```python
from build123d import *

# Parameters (mm, degrees)
SKETCH_1_W          = 403
SKETCH_1_H          = 40
EXTRUDE_1_DEPTH     = 2
CUT_EXTRUDE_1_DEPTH = 203.5
FILLET_1_R          = 1.5
SKETCH_3_R          = 2.1
SKETCH_3_R_2        = 1.6
SKETCH_3_R_3        = 2.6
CUT_EXTRUDE_2_DEPTH = 203.5


with BuildPart() as part:
    # 草图1 → 凸台-拉伸1 (new body)
    with BuildSketch(Plane.XY):
        Rectangle(SKETCH_1_W, SKETCH_1_H)
    extrude(amount=EXTRUDE_1_DEPTH)

    # 草图2 → 切除-拉伸1 (cut, through all)
    with BuildSketch(Plane.XY.offset(2)):
        Polygon((-157.550139231, -12), (-185, 8.270666414), (-185, -12), align=None)
        Polygon((-179.949860769, 12), (-155.5, -6.055281799), (-155.5, 12), align=None)
        Polygon((-149.5, 6.055281799), (-149.5, -12), (-125.050139231, -12), align=None)
        Polygon((-147.449860769, 12), (-123, -6.055281799), (-123, 12), align=None)
        Polygon((-87, 6.518202701), (-87, -12), (-58.06530828, -12), align=None)
        Polygon((-84.43469172, 12), (-55.5, -6.518202701), (-55.5, 12), align=None)
        Polygon((-46.93469172, 12), (-18, -6.518202701), (-18, 12), align=None)
        Polygon((-49.5, 6.518202701), (-49.5, -12), (-20.56530828, -12), align=None)
        Polygon((46.93469172, 12), (18, 12), (18, -6.518202701), align=None)
        Polygon((49.5, -12), (49.5, 6.518202701), (20.56530828, -12), align=None)
        Polygon((84.43469172, 12), (55.5, 12), (55.5, -6.518202701), align=None)
        Polygon((87, 6.518202701), (58.06530828, -12), (87, -12), align=None)
        Polygon((123, 12), (123, -6.055281799), (147.449860769, 12), align=None)
        Polygon((149.5, 6.055281799), (125.050139231, -12), (149.5, -12), align=None)
        Polygon((155.5, 12), (155.5, -6.055281799), (179.949860769, 12), align=None)
        Polygon((185, 8.270666414), (157.550139231, -12), (185, -12), align=None)
    extrude(amount=-CUT_EXTRUDE_1_DEPTH, mode=Mode.SUBTRACT)

    # 圆角1
    fillet_1_edges = [part.edges().sort_by_distance(p)[0] for p in [
        (-87, 6.518202701, 1),
        (-58.06530828, -12, 1),
        (-87, -12, 1),
        (149.5, 6.055281799, 1),
        (149.5, -12, 1),
        (125.050139231, -12, 1),
        (155.5, 12, 1),
        (179.949860769, 12, 1),
        (155.5, -6.055281799, 1),
        (185, 8.270666414, 1),
        (185, -12, 1),
        (157.550139231, -12, 1),
        (49.5, -12, 1),
        (20.56530828, -12, 1),
        (49.5, 6.518202701, 1),
        (84.43469172, 12, 1),
        (55.5, -6.518202701, 1),
        (55.5, 12, 1),
        (87, 6.518202701, 1),
        (87, -12, 1),
        (58.06530828, -12, 1),
        (123, 12, 1),
        (147.449860769, 12, 1),
        (123, -6.055281799, 1),
        (-157.550139231, -12, 1),
        (-185, -12, 1),
        (-185, 8.270666414, 1),
        (-84.43469172, 12, 1),
        (-55.5, 12, 1),
        (-55.5, -6.518202701, 1),
        (-46.93469172, 12, 1),
        (-18, 12, 1),
        (-18, -6.518202701, 1),
        (-49.5, 6.518202701, 1),
        (-20.56530828, -12, 1),
        (-49.5, -12, 1),
        (46.93469172, 12, 1),
        (18, -6.518202701, 1),
        (18, 12, 1),
        (-179.949860769, 12, 1),
        (-155.5, 12, 1),
        (-155.5, -6.055281799, 1),
        (-149.5, 6.055281799, 1),
        (-125.050139231, -12, 1),
        (-149.5, -12, 1),
        (-147.449860769, 12, 1),
        (-123, 12, 1),
        (-123, -6.055281799, 1),
    ]]
    fillet(fillet_1_edges, radius=FILLET_1_R)

    # 草图3 → 切除-拉伸2 (cut, through all)
    with BuildSketch(Plane(origin=(0, 0, 0), x_dir=(-1, 0, 0), z_dir=(0, 0, -1))):
        with Locations((195, -7.5)):
            Circle(SKETCH_3_R)
        with Locations((-195, 7.5)):
            Circle(SKETCH_3_R)
        with Locations((195, 7.5)):
            Circle(SKETCH_3_R)
        with Locations((105, 7.5)):
            Circle(SKETCH_3_R)
        with Locations((105, -7.5)):
            Circle(SKETCH_3_R)
        with Locations((-105, 7.5)):
            Circle(SKETCH_3_R)
        with Locations((-105, -7.5)):
            Circle(SKETCH_3_R)
        with Locations((-195, -7.5)):
            Circle(SKETCH_3_R)
        with Locations((-152.5, -14.5)):
            Circle(SKETCH_3_R_2)
        with Locations((-185, 14.5)):
            Circle(SKETCH_3_R_2)
        with Locations((-185, -14.5)):
            Circle(SKETCH_3_R_2)
        with Locations((185, -14.5)):
            Circle(SKETCH_3_R_2)
        with Locations((-52.5, -14.5)):
            Circle(SKETCH_3_R_2)
        with Locations((52.5, -14.5)):
            Circle(SKETCH_3_R_2)
        with Locations((152.5, -14.5)):
            Circle(SKETCH_3_R_2)
        with Locations((152.5, 14.5)):
            Circle(SKETCH_3_R_2)
        with Locations((185, 14.5)):
            Circle(SKETCH_3_R_2)
        with Locations((-152.5, 14.5)):
            Circle(SKETCH_3_R_2)
        with Locations((-52.5, 14.5)):
            Circle(SKETCH_3_R_2)
        with Locations((52.5, 14.5)):
            Circle(SKETCH_3_R_2)
        with Locations((0, -7.5)):
            Circle(SKETCH_3_R_3)
        with Locations((0, 7.5)):
            Circle(SKETCH_3_R_3)
        with BuildLine():
            Line((-57, 12), (-79.30828758, 12))
            ThreePointArc((-79.30828758, 12), (-80.7479248, 10.921241824), (-80.116868125, 9.236592899))
            Line((-80.116868125, 9.236592899), (-57.808580545, -5.040711152))
            ThreePointArc((-57.808580545, -5.040711152), (-56.279885709, -5.093144242), (-55.5, -3.777304051))
            Line((-55.5, -3.777304051), (-55.5, 10.5))
            ThreePointArc((-55.5, 10.5), (-55.939339828, 11.560660172), (-57, 12))
        make_face()
        with BuildLine():
            Line((-49.5, 3.777304051), (-49.5, -10.5))
            ThreePointArc((-49.5, -10.5), (-49.060660172, -11.560660172), (-48, -12))
            Line((-48, -12), (-25.69171242, -12))
            ThreePointArc((-25.69171242, -12), (-24.2520752, -10.921241824), (-24.883131875, -9.236592899))
            Line((-24.883131875, -9.236592899), (-47.191419455, 5.040711152))
            ThreePointArc((-47.191419455, 5.040711152), (-48.720114291, 5.093144242), (-49.5, 3.777304051))
        make_face()
        with BuildLine():
            Line((-157, 12), (-175.393541154, 12))
            ThreePointArc((-175.393541154, 12), (-176.818317426, 10.96905498), (-176.284605696, 9.2933501))
            Line((-176.284605696, 9.2933501), (-157.891064542, -4.289572599))
            ThreePointArc((-157.891064542, -4.289572599), (-156.324202994, -4.422063619), (-155.5, -3.082922698))
            Line((-155.5, -3.082922698), (-155.5, 10.5))
            ThreePointArc((-155.5, 10.5), (-155.939339828, 11.560660172), (-157, 12))
        make_face()
        with BuildLine():
            Line((-123, -3.082922698), (-123, 10.5))
            ThreePointArc((-123, 10.5), (-123.439339828, 11.560660172), (-124.5, 12))
            Line((-124.5, 12), (-142.893541154, 12))
            ThreePointArc((-142.893541154, 12), (-144.318317426, 10.96905498), (-143.784605696, 9.2933501))
            Line((-143.784605696, 9.2933501), (-125.391064542, -4.289572599))
            ThreePointArc((-125.391064542, -4.289572599), (-123.824202994, -4.422063619), (-123, -3.082922698))
        make_face()
        with BuildLine():
            Line((149.5, -10.5), (149.5, 3.082922698))
            ThreePointArc((149.5, 3.082922698), (148.675797006, 4.422063619), (147.108935458, 4.289572599))
            Line((147.108935458, 4.289572599), (128.715394304, -9.2933501))
            ThreePointArc((128.715394304, -9.2933501), (128.181682574, -10.96905498), (129.606458846, -12))
            Line((129.606458846, -12), (148, -12))
            ThreePointArc((148, -12), (149.060660172, -11.560660172), (149.5, -10.5))
        make_face()
        with BuildLine():
            Line((175.393541154, 12), (157, 12))
            ThreePointArc((157, 12), (155.939339828, 11.560660172), (155.5, 10.5))
            Line((155.5, 10.5), (155.5, -3.082922698))
            ThreePointArc((155.5, -3.082922698), (156.324202994, -4.422063619), (157.891064542, -4.289572599))
            Line((157.891064542, -4.289572599), (176.284605696, 9.2933501))
            ThreePointArc((176.284605696, 9.2933501), (176.818317426, 10.96905498), (175.393541154, 12))
        make_face()
        with BuildLine():
            Line((87, -10.5), (87, 3.777304051))
            ThreePointArc((87, 3.777304051), (86.220114291, 5.093144242), (84.691419455, 5.040711152))
            Line((84.691419455, 5.040711152), (62.383131875, -9.236592899))
            ThreePointArc((62.383131875, -9.236592899), (61.7520752, -10.921241824), (63.19171242, -12))
            Line((63.19171242, -12), (85.5, -12))
            ThreePointArc((85.5, -12), (86.560660172, -11.560660172), (87, -10.5))
        make_face()
        with BuildLine():
            Line((142.893541154, 12), (124.5, 12))
            ThreePointArc((124.5, 12), (123.439339828, 11.560660172), (123, 10.5))
            Line((123, 10.5), (123, -3.082922698))
            ThreePointArc((123, -3.082922698), (123.824202994, -4.422063619), (125.391064542, -4.289572599))
            Line((125.391064542, -4.289572599), (143.784605696, 9.2933501))
            ThreePointArc((143.784605696, 9.2933501), (144.318317426, 10.96905498), (142.893541154, 12))
        make_face()
        with BuildLine():
            Line((-161.215394304, -9.2933501), (-182.608935458, 6.504957214))
            ThreePointArc((-182.608935458, 6.504957214), (-184.175797006, 6.637448235), (-185, 5.298307314))
            Line((-185, 5.298307314), (-185, -10.5))
            ThreePointArc((-185, -10.5), (-184.560660172, -11.560660172), (-183.5, -12))
            Line((-183.5, -12), (-162.106458846, -12))
            ThreePointArc((-162.106458846, -12), (-160.681682574, -10.96905498), (-161.215394304, -9.2933501))
        make_face()
        with BuildLine():
            Line((79.30828758, 12), (57, 12))
            ThreePointArc((57, 12), (55.939339828, 11.560660172), (55.5, 10.5))
            Line((55.5, 10.5), (55.5, -3.777304051))
            ThreePointArc((55.5, -3.777304051), (56.279885709, -5.093144242), (57.808580545, -5.040711152))
            Line((57.808580545, -5.040711152), (80.116868125, 9.236592899))
            ThreePointArc((80.116868125, 9.236592899), (80.7479248, 10.921241824), (79.30828758, 12))
        make_face()
        with BuildLine():
            Line((41.80828758, 12), (19.5, 12))
            ThreePointArc((19.5, 12), (18.439339828, 11.560660172), (18, 10.5))
            Line((18, 10.5), (18, -3.777304051))
            ThreePointArc((18, -3.777304051), (18.779885709, -5.093144242), (20.308580545, -5.040711152))
            Line((20.308580545, -5.040711152), (42.616868125, 9.236592899))
            ThreePointArc((42.616868125, 9.236592899), (43.2479248, 10.921241824), (41.80828758, 12))
        make_face()
        with BuildLine():
            Line((182.608935458, 6.504957214), (161.215394304, -9.2933501))
            ThreePointArc((161.215394304, -9.2933501), (160.681682574, -10.96905498), (162.106458846, -12))
            Line((162.106458846, -12), (183.5, -12))
            ThreePointArc((183.5, -12), (184.560660172, -11.560660172), (185, -10.5))
            Line((185, -10.5), (185, 5.298307314))
            ThreePointArc((185, 5.298307314), (184.175797006, 6.637448235), (182.608935458, 6.504957214))
        make_face()
        with BuildLine():
            Line((-62.383131875, -9.236592899), (-84.691419455, 5.040711152))
            ThreePointArc((-84.691419455, 5.040711152), (-86.220114291, 5.093144242), (-87, 3.777304051))
            Line((-87, 3.777304051), (-87, -10.5))
            ThreePointArc((-87, -10.5), (-86.560660172, -11.560660172), (-85.5, -12))
            Line((-85.5, -12), (-63.19171242, -12))
            ThreePointArc((-63.19171242, -12), (-61.7520752, -10.921241824), (-62.383131875, -9.236592899))
        make_face()
        with BuildLine():
            Line((-128.715394304, -9.2933501), (-147.108935458, 4.289572599))
            ThreePointArc((-147.108935458, 4.289572599), (-148.675797006, 4.422063619), (-149.5, 3.082922698))
            Line((-149.5, 3.082922698), (-149.5, -10.5))
            ThreePointArc((-149.5, -10.5), (-149.060660172, -11.560660172), (-148, -12))
            Line((-148, -12), (-129.606458846, -12))
            ThreePointArc((-129.606458846, -12), (-128.181682574, -10.96905498), (-128.715394304, -9.2933501))
        make_face()
        with BuildLine():
            Line((-19.5, 12), (-41.80828758, 12))
            ThreePointArc((-41.80828758, 12), (-43.2479248, 10.921241824), (-42.616868125, 9.236592899))
            Line((-42.616868125, 9.236592899), (-20.308580545, -5.040711152))
            ThreePointArc((-20.308580545, -5.040711152), (-18.779885709, -5.093144242), (-18, -3.777304051))
            Line((-18, -3.777304051), (-18, 10.5))
            ThreePointArc((-18, 10.5), (-18.439339828, 11.560660172), (-19.5, 12))
        make_face()
        with BuildLine():
            Line((49.5, -10.5), (49.5, 3.777304051))
            ThreePointArc((49.5, 3.777304051), (48.720114291, 5.093144242), (47.191419455, 5.040711152))
            Line((47.191419455, 5.040711152), (24.883131875, -9.236592899))
            ThreePointArc((24.883131875, -9.236592899), (24.2520752, -10.921241824), (25.69171242, -12))
            Line((25.69171242, -12), (48, -12))
            ThreePointArc((48, -12), (49.060660172, -11.560660172), (49.5, -10.5))
        make_face()
    extrude(amount=-CUT_EXTRUDE_2_DEPTH, mode=Mode.SUBTRACT)


solid = part.part
```
Work out the finished part from the listing and answer in its coordinate system (mm). A direction names the side the tool comes from. Round coordinates to 2 decimals unless told otherwise and drop trailing zeros. Return JSON: item names as keys, results as strings. Group by question number.
Q1. For faces 3 (the flat face through (73.69, -2, 1.01)), 4 (the flat face through (-3, 0, 2)), determine the directions among +Z, -Z, +X, -X, +Y, -Y from which every point of the face is accessible in a straight line to the end or side of a thin tool.
Q2. The part is cut by section A-A on z = 0.6. Count the separate pieces of the cut face and the enclosed holes in it, then the cut area to 3 significant figures.
Q3. Find the intervals of material crossed by L1, parallel to Y at x = 105, z = 1.4; L2, parallel to Y at x = 52.5, z = 1.4; L3, parallel to Y at x = 158, z = 1, in increasing order.
Q4. The mould has two halves that part along X. Classify faces 1 (the flat face through (-35.88, -2.2, 1.01)), 2 (the flat face through (-3, 0, 0)): released by +X, released by -X, zero draft, split by the parting line, or undercut.
Solved:
{
 "1": {"face 3": "+Z, -Z", "face 4": "+Z, +X, -X, +Y, -Y"},
 "2": {"separate pieces": "1", "enclosed holes": "38", "area": "12,000 mm²"},
 "3": {"L1": "-20 to -9.6, -5.4 to 5.4, 9.6 to 20", "L2": "-20 to -16.1, -12.9 to 12.9, 16.1 to 20", "L3": "-20 to -4.21, 12 to 20"},
 "4": {"face 1": "undercut", "face 2": "zero draft"}
}
